Autodesk Inventor part; units mm, degrees
ref_plane "Work Plane4" through (0, 4, -25) normal (0, 0.5487, -0.836) x (-1, 0, 0)
ref_plane "YZ Plane" through (0, 0, 0) normal (1, 0, 0) x (0, 1, 0)
ref_plane "XZ Plane" through (0, 0, 0) normal (0, 1, 0) x (-1, 0, 0)
sketch "Sketch7" plane through (0, 0, 0) normal (1, 0, 0) x (0, 1, 0)
  line L0 (36, 0) -> (36, -4)
  line L1 (36, -4) -> (4, -25)
  line L2 (4, -25) -> (0, -25)
  line L3 (0, -25) -> (0, 0)
  line L4 (0, 0) -> (36, 0)
  line L5 (36, -4) -> (16.6104, -4)
  line L6 (4, -7.9408) -> (4, -25)
  line L7 (16, 0) -> (0, -5)
  line L8 (4, -7.9408) -> (16.6104, -4)
  dimension "d35" = 4
  dimension "d36" = 25
  dimension "d37" = 36
  dimension "d43" = 4
  dimension "d44" = 20
  dimension "d45" = 20
extrude "Extrusion6" add sketch "Sketch7" along normal mid plane 54 contours L0 L5 L8 L6 L2 L3 L7 L4
sketch "Sketch8" plane through (27, 36, -4) normal (0, 0, -1) x (-1, 0, 0)
  line L0 (0, -10) -> (13.5, -10) construction
  line L1 (13.5, -10) -> (27, -10) construction
  line L2 (27, -10) -> (40.5, -10) construction
  line L3 (40.5, -10) -> (54, -10) construction
  circle A0 centre (13.5, -10) radius 2.65
  circle A1 centre (40.5, -10) radius 2.65
  line L4 (0, -19.3896) -> (0, 0)
  line L5 (54, 0) -> (54, -19.3896)
  line L6 (54, 0) -> (0, 0)
  point P0 (27, -36)
  dimension "d46" = 5.3
  dimension "d55" = 10
extrude "Extrusion7" cut sketch "Sketch8" against normal through all
sketch "Sketch9" plane through (-27, 4, -7.9408) normal (0, 1, 0) x (1, 0, 0)
  line L0 (54, 17.0592) -> (54, 0)
  line L1 (54, 7.0592) -> (40.5, 7.0592) construction
  line L2 (40.5, 7.0592) -> (27, 7.0592) construction
  line L3 (27, 7.0592) -> (13.5, 7.0592) construction
  line L4 (13.5, 7.0592) -> (0, 7.0592) construction
  line L5 (0, 0) -> (0, 17.0592)
  circle A0 centre (40.5, 7.0592) radius 2.65
  circle A1 centre (13.5, 7.0592) radius 2.65
  line L6 (54, 17.0592) -> (0, 17.0592)
  point P0 (27, -7.9408)
  dimension "d49" = 5.3
  dimension "d56" = 10
  dimension "d57" = 27
extrude "Extrusion8" cut sketch "Sketch9" against normal blind 10
ref_plane "Work Plane4" through (0, 4, -25) normal (0, 0.5487, -0.836) x (-1, 0, 0)
sketch "Sketch10" plane through (0, 4, -25) normal (0, 0.5487, -0.836) x (-1, 0, 0)
  line L0 (-27, 38.2753) -> (-25, 38.2753)
  line L1 (-25, 38.2753) -> (-25, 0)
  line L2 (-25, 0) -> (-27, 0)
  line L3 (-27, 0) -> (-27, 38.2753)
  line L4 (27, 0) -> (25, 0)
  line L5 (25, 0) -> (25, 38.2753)
  line L6 (25, 38.2753) -> (27, 38.2753)
  line L7 (27, 38.2753) -> (27, 0)
  line L8 (-1, 38.2753) -> (1, 38.2753)
  line L9 (1, 38.2753) -> (1, 0)
  line L10 (1, 0) -> (-1, 0)
  line L11 (-1, 0) -> (-1, 38.2753)
  line L12 (27, 38.2753) -> (-27, 38.2753)
  line L13 (-27, 0) -> (27, 0)
  point P0 (0, 10.3722)
  point P1 (0, 38.2753)
  dimension "d52" = 2
extrude "Extrusion9" add sketch "Sketch10" against normal up to next contours L0 L1 L2 L3 | L8 L9 L10 L11 | L6 L7 L4 L5
equation "\"BendRadius\" = Thickness"
equation "\"BendReliefWidth\" = Thickness"
equation "\"BendReliefDepth\" = 0.5 * Thickness"
equation "\"CornerReliefSize\" = 4 * Thickness"
equation "\"MinimumRemnant\" = 2 * Thickness"
equation "\"TransitionRadius\" = BendRadius"
equation "\"JacobiRadiusSize\" = Thickness"
equation "\"GapSize\" = Thickness"
properties part number "Soporte Cajas" material "Rubber"
Build history of the part. All positions in model axes, mm. A direction names the side the tool comes from. Round coordinates to 2 decimals unless told otherwise and drop trailing zeros. Loops run counter-clockwise (first coordinate to the right, second up) from the corner with the lowest first, then second, coordinate; pieces in that order, holes last. Notation, with made-up numbers: (52, -0.5) -> (104, -0.5) arc R8 ccw to (104, 10.5) -> close; hole circle Ø2 at (64.25, -20.5). An arc over 180 degrees is marked (long way). Answer in a Markdown table with one row per item.
Item 1: Drill centre lines: L1, parallel to X at y = 1.15, z = -15; L2, parallel to X at y = 15, z = -17.25; L3, parallel to Z at x = 16, y = 32. Where is each one in solid material? Low to high. Write a range as [from, to].
Answers below:
| item | result |
|---|---|
| L1 | x = [-27, -16.15], [-10.85, 10.85], [16.15, 27] |
| L2 | x = [-27, -25], [-1, 1], [25, 27] |
| L3 | z = [-4, 0] |
Item 2: Which spindle directions (+Z, -Z, +X, -X, +Y, -Y) get a long thin tool onto all of the face, cutting with end or side? Do faces 1 (the flat face through (-0.378, 8.112, -2.465)), 2 (the flat face through (-1, 14, -12)). Say none if no direction does.
Answers below:
| item | result |
|---|---|
| face 1 | +Z, +X, -X, -Y |
| face 2 | -Z, +Y |
Item 3: Pin check, flat tips, straight feed: pin 1 (9.5 mm diameter, centred on x = -9, y = 30.5, fed in from -Z); pin 2 (5 mm diameter, centred on x = 18.5, z = -17.5, fed in from +Y); pin 3 (3 mm diameter, centred on x = 14.5, y = 15.5, fed in from -Z). Stop position of each tip, or through.
Answers below:
| item | result |
|---|---|
| pin 1 | stops at z = -4 |
| pin 2 | stops at y = 4 |
| pin 3 | stops at z = -4.82 |
Item 4: Saw through at B-B (y = 27). Write the cut outline in (x, z), and give its area (3 significant figures).
Answers below:
| item | result |
|---|---|
| outline | (-27, -9.9) -> (-25, -9.9) -> (-25, -4) -> (-15.95, -4) -> (-15.95, 0) -> (-27, 0) -> close; (-11.05, -4) -> (-1, -4) -> (-1, -9.9) -> (1, -9.9) -> (1, -4) -> (11.05, -4) -> (11.05, 0) -> (-11.05, 0) -> close; (15.95, -4) -> (25, -4) -> (25, -9.9) -> (27, -9.9) -> (27, 0) -> (15.95, 0) -> close |
| area | 212 mm² |
Item 5: Mould opens along X. For faces 3 (the flat face through (0, 36, -2)), 4 (the flat face through (1, 17, -10)), 5 (the flat face through (27, 14, -10)) say: +X half, -X half, draft (parallel to the pull), parting line (faces both ways), or undercut.
Answers below:
| item | result |
|---|---|
| face 3 | draft |
| face 4 | undercut |
| face 5 | +X half |
Item 6: Saw through at C-C (z = -15). Write the cut outline in (x, y).
Answers below:
| item | result |
|---|---|
| outline | (-27, 0) -> (-16.15, 0) -> (-16.15, 4) -> (-25, 4) -> (-25, 19.24) -> (-27, 19.24) -> close; (-10.85, 0) -> (10.85, 0) -> (10.85, 4) -> (1, 4) -> (1, 19.24) -> (-1, 19.24) -> (-1, 4) -> (-10.85, 4) -> close; (16.15, 0) -> (27, 0) -> (27, 19.24) -> (25, 19.24) -> (25, 4) -> (16.15, 4) -> close |
Item 7: Saw through at A-A (x = -13.5). Write the cut outline in (y, z).
Answers below:
| item | result |
|---|---|
| outline | (0, -25) -> (4, -25) -> (4, -17.65) -> (0, -17.65) -> close; (0, -12.35) -> (4, -12.35) -> (4, -7.94) -> (16.61, -4) -> (23.35, -4) -> (23.35, 0) -> (16, 0) -> (0, -5) -> close; (28.65, -4) -> (36, -4) -> (36, 0) -> (28.65, 0) -> close |
Item 8: Saw through at D-D (x = -23.5). Write the cut outline in (y, z), and give its area (3 significant figures).
Answers below:
| item | result |
|---|---|
| outline | (0, -25) -> (4, -25) -> (4, -7.94) -> (16.61, -4) -> (36, -4) -> (36, 0) -> (16, 0) -> (0, -5) -> close |
| area | 213 mm² |
